Design review of the part shown in the three views and the two pictorial views. Dimensions are in mm from the part's minimum x, y and z. A direction names the side the tool comes from. Coordinates: 2 decimals unless noted, no trailing zeros. Loops run counter-clockwise (first coordinate to the right, second up) from the corner with the lowest first, then second, coordinate; pieces in that order, holes last.
Q1. Add section A-A on x = 34. Give the boundary of the cut face in (y, z).
Q2. Machinability: for the marked faces 1, 2 and 3, which of the approach directions +Z, -Z, +X, -X, +Y, -Y give a long, thin tool a straight path to every point of the face, cutting with its end or side? Answer none if there is none.
Q3. Add section D-D on y = 16.5. Give the boundary of the cut face in (x, z), and give its area (3 significant figures).
Q4. Wall thickness on probe 1 along X at (y, z) = (10, 18); probe 2 along X at (y, z) = (13.75, 36); probe 3 along Z at (x, y) = (7, 2.5): over which ranges is each line inside the solid? List them lowest first.
Q5. For P1, Ø9, axis at x = 7, y = 10, coming from the -Z side; P2, Ø1.5, axis at y = 15, z = 7.5, coming from the +X side; P3, Ø3.5, axis at x = 7, z = 36, coming from the -Y side; P4, Ø2.5, axis at x = 1, y = 13, coming from the -Z side, all flat-tipped, find the tip position at first contact; note any pin that passes through.
Q6. Add section B-B on z = 29. Give the boundary of the cut face in (x, y), and give its area (3 significant figures).
Q7. Draft analysis for pull direction Z (two halves, no side actions). For the marked faces 4, 5 and 6, state which applies: released by +Z, released by -Z, zero draft, split by the parting line, or undercut.
Q8. Add section C-C on x = 53. Give the boundary of the cut face in (y, z), and give its area (3 significant figures).
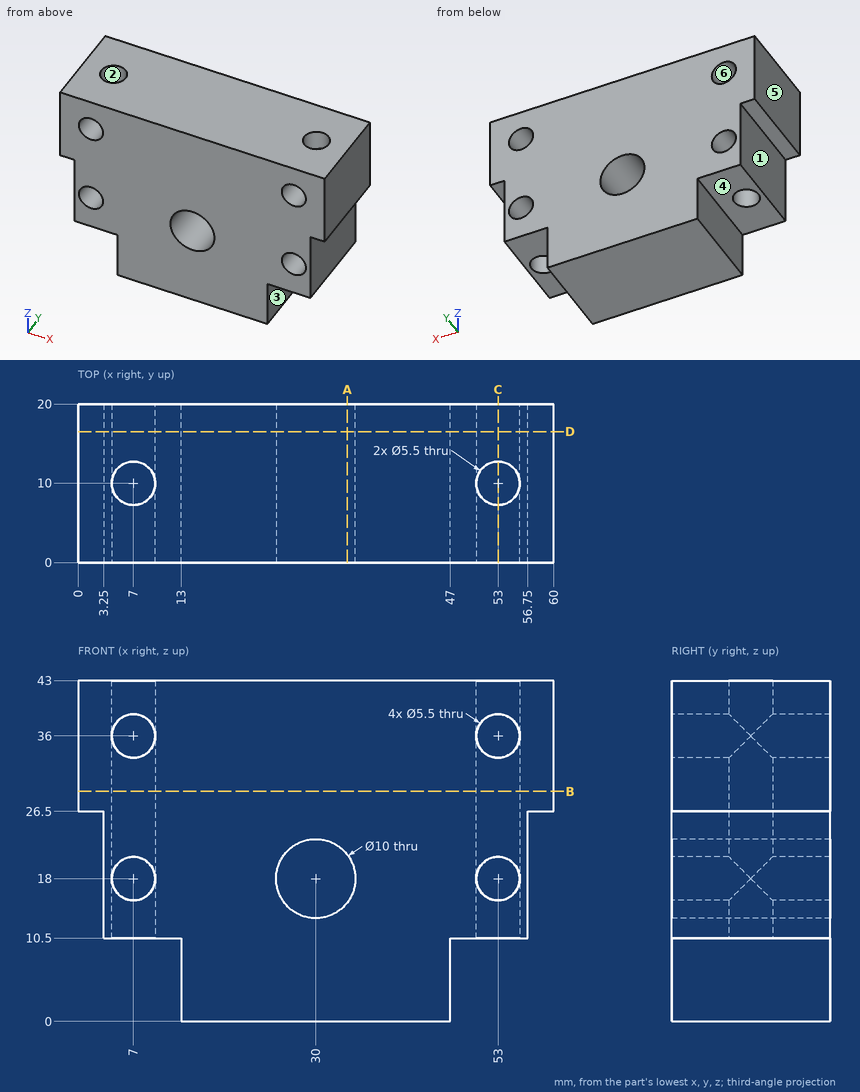
Entries:
1. outline: (0, 0) - (20, 0) - (20, 15) - (0, 15) - close; (0, 21) - (20, 21) - (20, 43) - (0, 43) - close
2. face 1: -Z, -X, +Y, -Y
2. face 2: +Z, -Z
2. face 3: -Z, +X, +Y, -Y
3. outline: (0, 26.5) - (3.25, 26.5) - (3.25, 10.5) - (13, 10.5) - (13, 0) - (47, 0) - (47, 10.5) - (56.75, 10.5) - (56.75, 26.5) - (60, 26.5) - (60, 43) - (0, 43) - close; hole circle Ø5.5 at (7, 18); hole circle Ø5.5 at (7, 36); hole circle Ø10 at (30, 18); hole circle Ø5.5 at (53, 18); hole circle Ø5.5 at (53, 36)
3. area: 2,030 mm2
4. probe 1: x = 3.25 to 4.25, 9.75 to 25, 35 to 50.25, 55.75 to 56.75
4. probe 2: x = 0 to 4.25, 9.75 to 50.25, 55.75 to 60
4. probe 3: z = 10.5 to 15.25, 20.75 to 33.25, 38.75 to 43
5. P1: stops at z = 10.5
5. P2: stops at x = 47
5. P3: passes through
5. P4: stops at z = 26.5
6. outline: (0, 0) - (60, 0) - (60, 20) - (0, 20) - close; hole circle Ø5.5 at (7, 10); hole circle Ø5.5 at (53, 10)
6. area: 1,150 mm2
7. face 4: released by -Z
7. face 5: zero draft
7. face 6: undercut
8. outline: (0, 10.5) - (7.25, 10.5) - (7.25, 15.25) - (0, 15.25) - close; (0, 20.75) - (7.25, 20.75) - (7.25, 33.25) - (0, 33.25) - close; (0, 38.75) - (7.25, 38.75) - (7.25, 43) - (0, 43) - close; (12.75, 10.5) - (20, 10.5) - (20, 15.25) - (12.75, 15.25) - close; (12.75, 20.75) - (20, 20.75) - (20, 33.25) - (12.75, 33.25) - close; (12.75, 38.75) - (20, 38.75) - (20, 43) - (12.75, 43) - close
8. area: 312 mm2
